Autodesk Inventor part; units mm, degrees
ref_plane "YZ Plane" through (0, 0, 0) normal (1, 0, 0) x (0, 1, 0)
ref_plane "XZ Plane" through (0, 0, 0) normal (0, 1, 0) x (-1, 0, 0)
ref_plane "XY Plane" through (0, 0, 0) normal (0, 0, 1) x (1, 0, 0)
sketch "Sketch1" plane through (0, 0, 0) normal (0, 1, 0) x (-1, 0, 0)
  line L0 (0.53, 20.25) -> (-28.77, 20.25)
  line L1 (-28.77, 20.25) -> (-28.77, -20.25)
  line L2 (-28.77, -20.25) -> (0.53, -20.25)
  line L3 (0.53, -20.25) -> (0.53, 20.25)
  point P0 (0, 0)
  dimension "d0" = 40.5
  dimension "d1" = 29.3
  dimension "d2" = -0.53
  dimension "d3" = 20.25
extrude "Plate1" add sketch "Sketch1" along normal blind 1.5
sketch "Sketch2" plane through (28.77, 0, 21.75) normal (0, 0, -1) x (-1, 0, 0)
  line L0 (29.3, 0) -> (0, 0)
  line L1 (0, 0) -> (0, 28.14)
  line L2 (0, 28.14) -> (29.3, 28.14)
  line L3 (29.3, 28.14) -> (29.3, 0)
edge flange "Flange1" height 28.14 angle 90 thickness 1.5 bend radius 0.31 thickness toward (0, 0, -1) relief tear relief width 1.5 relief depth 0.75 corner gap 0.31 corner form 0 edges at (14.12, 1.5, 20.25) (14.12, 1.5, -20.25) wall of the first edge with corners at (-0.53, 0, 21.75) (28.77, 0, 21.75) (28.77, 28.14, 21.75) (-0.53, 28.14, 21.75)
bend "Bend1"
corner "Corner1"
sketch "Sketch6" plane through (-0.53, 28.14, 21.75) normal (0, 0, 1) x (1, 0, 0)
  point P0 (0.53, -28.14)
sketch "Sketch8" plane through (28.77, 28.14, -21.75) normal (0, 0, -1) x (-1, 0, 0)
  circle A0 centre (2.5, -2.545) radius 0.7835
  circle A1 centre (2.5, -17.595) radius 0.7835
  circle A2 centre (17.6, -2.545) radius 0.7835
  circle A3 centre (17.6, -17.595) radius 0.7835
  circle A4 centre (37.6, -2.545) radius 0.7835
  circle A5 centre (37.6, -17.595) radius 0.7835
  point P0 (28.77, -28.14)
hole "Hole4" at (26.27, 25.595, -21.75) at (26.27, 10.545, -21.75) at (11.17, 25.595, -21.75) at (11.17, 10.545, -21.75) at (-8.83, 25.595, -21.75) at (-8.83, 10.545, -21.75) direction (0, 0, 1) diameter 2.1 depth 1.5
sketch "Sketch9" plane through (28.77, 28.14, -21.75) normal (0, 0, -1) x (-1, 0, 0)
  circle A0 centre (30.1, -10.07) radius 6
  point P0 (28.77, -28.14)
sketch "Sketch10" plane through (-0.53, 28.14, 21.75) normal (0, 0, 1) x (1, 0, 0)
  point P0 (0.53, -28.14)
sketch "Sketch11" plane through (-0.53, 28.14, 21.75) normal (0, 0, 1) x (1, 0, 0)
  point P0 (0.53, -28.14)
sketch "Sketch15" plane through (0, 0, 0) normal (0, -1, 0) x (1, 0, 0)
  point P0 (0, 0)
sketch "Sketch16" plane through (0, 0, 0) normal (0, -1, 0) x (1, 0, 0)
  circle A0 centre (6.47, 14.94) radius 1.55
  line L0 (28.77, 19.94) -> (-0.53, 19.94)
  line L1 (-0.53, -19.94) -> (-0.53, 19.94)
  circle A1 centre (21.77, 14.94) radius 1.55
  line L2 (28.77, 19.94) -> (28.77, -19.94)
  circle A2 centre (6.47, 4.8) radius 1.55
  circle A3 centre (21.77, 4.8) radius 1.55
  point P0 (0, 0)
  dimension "d65" = 3.1
  dimension "d66" = 5
  dimension "d67" = 7
  dimension "d68" = 3.1
  dimension "d69" = 5
  dimension "d70" = 7
  dimension "d71" = 3.1
  dimension "d72" = 15.14
  dimension "d73" = 7
  dimension "d74" = 3.1
  dimension "d75" = 15.14
  dimension "d76" = 7
extrude "Cut6" cut sketch "Sketch16" against normal blind 1.5
sketch "Sketch18" plane through (-0.53, 28.14, 21.75) normal (0, 0, 1) x (1, 0, 0)
  circle A0 centre (-0.8, -10.07) radius 6
  point P0 (0.53, -28.14)
fillet "Corner Round1" radius 1 4 edges at (-0.53, 28.14, -21) (28.77, 28.14, -21) (28.77, 28.14, 21) (-0.53, 28.14, 21)
sketch "Sketch19" plane through (-0.53, 1.81, 21.75) normal (0, 0, 1) x (1, 0, 0)
  circle A0 centre (6.1, 24.26) radius 0.7835
  circle A1 centre (19.32, 23.26) radius 0.7835
  circle A2 centre (26.62, 16.26) radius 0.7835
  circle A3 centre (19.32, 9.26) radius 0.7835
  circle A4 centre (6.1, 8.26) radius 0.7835
  point P0 (0.53, -1.81)
hole "Hole6" at (5.57, 26.07, 21.75) at (18.79, 25.07, 21.75) at (26.09, 18.07, 21.75) at (18.79, 11.07, 21.75) at (5.57, 10.07, 21.75) direction (0, 0, -1) diameter 2.1 depth 1.5
hole "Hole7" at (-1.33, 18.07, 21.75) direction (0, 0, -1) diameter 13.5 depth 1.5
hole "Hole8" at (-1.33, 18.07, -21.75) direction (0, 0, 1) diameter 13.5 depth 1.5
equation "\"d55\" = Thickness"
equation "\"d77\" = Thickness"
equation "\"d94\" = Thickness"
equation "\"d101\" = Thickness"
equation "\"d108\" = Thickness"
equation "\"d4\" = Thickness"
equation "\"d5\" = BendReliefWidth"
equation "\"d6\" = BendReliefDepth"
equation "\"d7\" = MinimumRemnant"
equation "\"d8\" = TransitionRadius"
equation "\"d11\" = BendRadius"
equation "\"d12\" = CornerReliefSize"
equation "\"d13\" = GapSize"
equation "\"d14\" = JacobiRadiusSize"
equation "\"BendReliefWidth\" = Thickness"
equation "\"BendReliefDepth\" = 0.5 * Thickness"
equation "\"CornerReliefSize\" = 4 * Thickness"
equation "\"MinimumRemnant\" = 2 * Thickness"
equation "\"TransitionRadius\" = BendRadius"
equation "\"JacobiRadiusSize\" = BendRadius"
equation "\"GapSize\" = Thickness"
properties part number "axis_25_bottom_frame" material "Aluminum 6061-AHC"
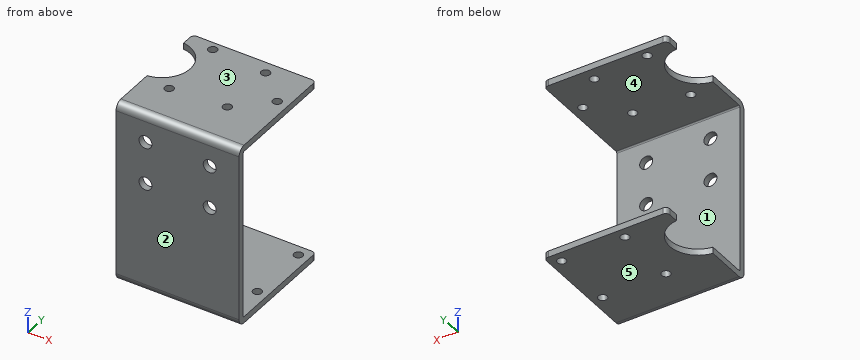
Can you work these out from the model? Positions are in its coordinate system, mm. Face numbers are marked on the shaded views. A direction names the side the tool comes from. Round coordinates to 2 decimals unless told otherwise and drop trailing zeros. Loops run counter-clockwise (first coordinate to the right, second up) from the corner with the lowest first, then second, coordinate; pieces in that order, holes last. Notation, with made-up numbers: (8.25, 43.25) - (46.25, 43.25) arc R18 cw to (46.25, 78.25) - close; hole circle Ø1 at (-3.5, -26.75). An arc over 180 degrees is marked (long way). Write item = value, one per line. Start each with the question number.
(1) If we section it at C-C (z = 14.94): Please give me the cut outline in (x, y), and give its area (4 significant figures).
(2) If we section it at D-D (x = 1.25): Please give me the cut outline in (y, z), and give its area (3 significant figures).
(3) For P1, Ø1.9, axis at x = 18.79, y = 25.07, coming from the +Z side; P2, Ø4, axis at x = 6.47, z = 4.8, coming from the +Y side; P3, Ø2.5, axis at x = 21.77, z = 14.94, coming from the +Y side, each with a flat end and sliding along its axis, tell me the tip position at first contact or that it passes through.
(4) If we mould it in two halves opening along Z, with no side actions, what happens to the marked faces 3, 4 and 5? For each: released by +Z, released by -Z, zero draft, split by the parting line, or undercut.
(5) For the marked faces 1 and 2, which set-ups out of +Z, -Z, +X, -X, +Y, -Y let a thin tool reach every point of the face, with its end or its side?
(6) If we section it at B-B (x = 18.79): Please give me the cut outline in (y, z), and give its area (3 significant figures).
(7) If we section it at A-A (y = 18.07): Please give me the cut outline in (x, z), and give its area (3 significant figures).
(8) If I drill on probe 1 along Z at (x, y) = (15.25, 17.25); probe 2 along Y at (x, z) = (5.57, 20.8); probe 3 along Y at (x, z) = (12, -3), over which ranges is the centre line in solid material (lowest first)? Write a range as [from, to].
Ans:
q1.outline = (-0.53, 0) - (4.92, 0) - (4.92, 1.5) - (-0.53, 1.5) - close; (8.02, 0) - (20.22, 0) - (20.22, 1.5) - (8.02, 1.5) - close; (23.32, 0) - (28.77, 0) - (28.77, 1.5) - (23.32, 1.5) - close
q1.area = 34.65 mm²
q2.outline = (0, -19.94) arc R1.81 ccw to (1.81, -21.75) - (11.83, -21.75) - (11.83, -20.25) - (1.81, -20.25) arc R0.31 cw to (1.5, -19.94) - (1.5, 19.94) arc R0.31 cw to (1.81, 20.25) - (11.83, 20.25) - (11.83, 21.75) - (1.81, 21.75) arc R1.81 ccw to (0, 19.94) - close; (24.31, -21.75) - (28.14, -21.75) - (28.14, -20.25) - (24.31, -20.25) - close; (24.31, 20.25) - (28.14, 20.25) - (28.14, 21.75) - (24.31, 21.75) - close
q2.area = 106 mm²
q3.P1 = -20.25
q3.P2 = 1.5
q3.P3 = through
q4.face_3 = released by +Z
q4.face_4 = undercut
q4.face_5 = released by -Z
q5.face_1 = +X, -X, +Y
q5.face_2 = +Z, -Z, +X, -X, -Y
q6.outline = (0, -19.94) arc R1.81 ccw to (1.81, -21.75) - (28.14, -21.75) - (28.14, -20.25) - (1.81, -20.25) arc R0.31 cw to (1.5, -19.94) - (1.5, 19.94) arc R0.31 cw to (1.81, 20.25) - (10.02, 20.25) - (10.02, 21.75) - (1.81, 21.75) arc R1.81 ccw to (0, 19.94) - close; (12.12, 20.25) - (24.02, 20.25) - (24.02, 21.75) - (12.12, 21.75) - close; (26.12, 20.25) - (28.14, 20.25) - (28.14, 21.75) - (26.12, 21.75) - close
q6.area = 138 mm²
q7.outline = (5.42, -21.75) - (28.77, -21.75) - (28.77, -20.25) - (5.42, -20.25) - close; (5.42, 20.25) - (25.04, 20.25) - (25.04, 21.75) - (5.42, 21.75) - close; (27.14, 20.25) - (28.77, 20.25) - (28.77, 21.75) - (27.14, 21.75) - close
q7.area = 66.9 mm²
q8.probe_1 = [-21.75, -20.25], [20.25, 21.75]
q8.probe_2 = [0.22, 9.02], [11.12, 25.02], [27.12, 28.14]
q8.probe_3 = [0, 1.5]
